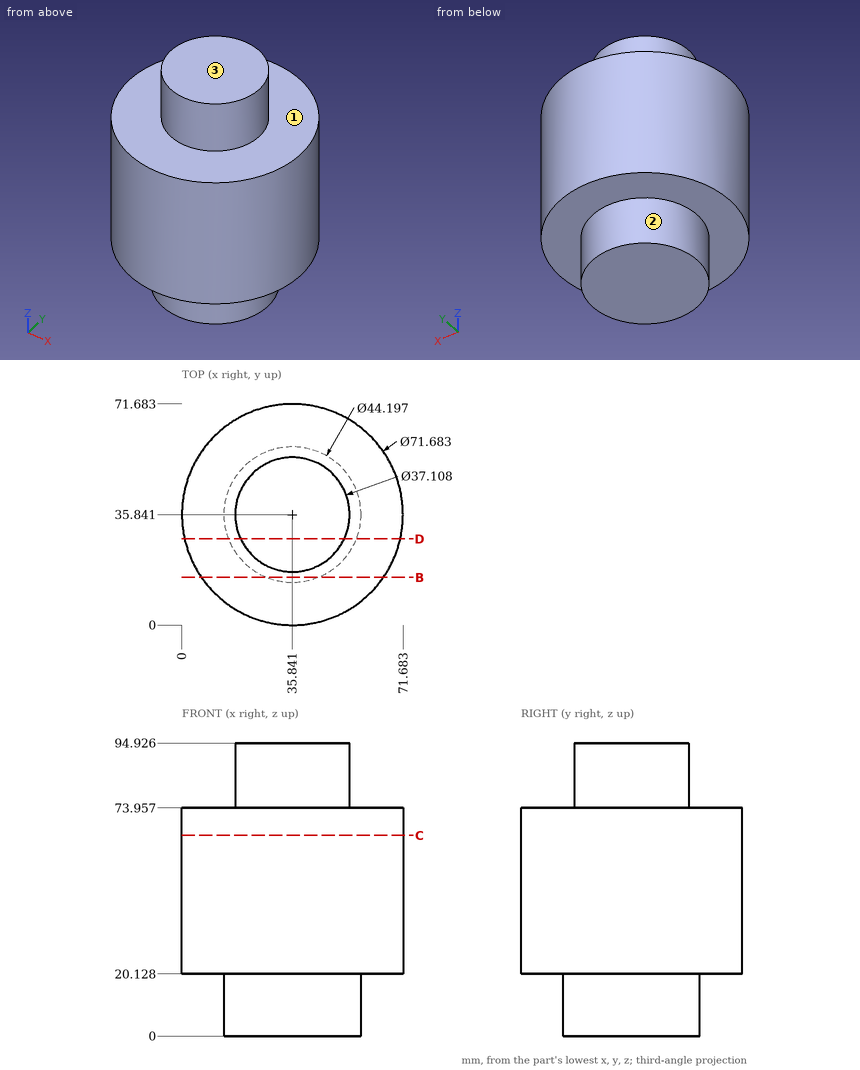
Here's the drawing with two shaded views (mm, measured from the low corner). I have some questions. A direction names the side the tool comes from. Give positions to 0.01 mm unless a question says otherwise; leave off trailing zeros. Write each loop counter-clockwise with the first axis right and the second up, starting at its lowest first coordinate (ties: lowest second). Pieces come first, ordered by that corner, then holes. Notation, with made-up numbers: (65.5, 40) -> (80.5, 40) arc R17 cw to (80.5, 45) -> close; hole circle Ø8 at (57, 11.25). An arc over 180 degrees is marked (long way). Use one line per item in the form item = value.
1) If I drill on L1, parallel to Z at x = 7, y = 36; L2, parallel to Y at x = 7, z = 49 (1 decimal); L3, parallel to Z at x = 25.5, y = 55, over which ranges is the centre line in solid material (lowest first)? Write a range as [from, to].
Verdict:
L1 = [20.13, 73.96]
L2 = [14.6, 57.1]
L3 = [0, 73.96]
2) Suppose I cut it at B-B (y = 15.5). Please give me the cut outline in (x, z) (1 decimal).
Verdict:
outline = (6.3, 20.1) -> (27.2, 20.1) -> (27.2, 0) -> (44.5, 0) -> (44.5, 20.1) -> (65.4, 20.1) -> (65.4, 74) -> (6.3, 74) -> close
3) Suppose I cut it at D-D (y = 28). Please give me the cut outline in (x, z) (1 decimal), and give its area (3 significant figures).
Verdict:
outline = (0.9, 20.1) -> (15.2, 20.1) -> (15.2, 0) -> (56.5, 0) -> (56.5, 20.1) -> (70.8, 20.1) -> (70.8, 74) -> (52.7, 74) -> (52.7, 94.9) -> (19, 94.9) -> (19, 74) -> (0.9, 74) -> close
area = 5,300 mm2
4) I'm going to push flat-ended pins straight in: pin 1 (5 mm diameter, centred on x = 41.5, y = 43.5, fed in from -Z); pin 2 (4 mm diameter, centred on x = 52, z = 15.5, fed in from +Y); pin 3 (12 mm diameter, centred on x = 53.5, z = 73.5, fed in from -Y); pin 4 (12 mm diameter, centred on y = 20.5, z = 63, fed in from +X). Where does each tip first touch, or does it pass through?
Verdict:
pin_1 = 0
pin_2 = 52.81
pin_3 = 1.95
pin_4 = 70.44
5) Suppose I cut it at C-C (z = 65). Please give me the cut outline in (x, y).
Verdict:
outline = circle Ø71.68 at (35.84, 35.84)
6) On a 3-axis mill with a long thin cutter (end or side, diameter ignored), from which of +Z, -Z, +X, -X, +Y, -Y can I reach the whole of each face in a straight line? I mean the marked faces 1, 2 and 3. Say none if no direction works.
Verdict:
face_1 = +Z
face_2 = -Z
face_3 = +Z, +X, -X, +Y, -Y
